from build123d import *

# Parameters (mm, degrees)
BOSS_EXTRUDE1_DEPTH = 6.35
SKETCH2_R           = 17.4625
SKETCH2_R_2         = 2.54
CUT_EXTRUDE1_DEPTH  = 706.764721773


with BuildPart() as part:
    # Sketch1 → Boss-Extrude1 (new body)
    with BuildSketch(Plane(origin=(0, 0, 0), x_dir=(0, 0, -1), z_dir=(1, 0, 0))):
        Polygon((0, 0), (0, 609.6), (50.8, 609.6), (355.6, 50.8), (355.6, 0), align=None)
        with BuildLine():
            Line((76.2, 101.6), (76.2, 357.336122773))
            ThreePointArc((76.2, 357.336122773), (95.323978482, 381.948549591), (123.898547552, 369.498966892))
            Line((123.898547552, 369.498966892), (263.390978155, 113.762844119))
            ThreePointArc((263.390978155, 113.762844119), (262.933861882, 88.634203469), (241.092430603, 76.2))
            Line((241.092430603, 76.2), (101.6, 76.2))
            ThreePointArc((101.6, 76.2), (83.639487758, 83.639487758), (76.2, 101.6))
        make_face(mode=Mode.SUBTRACT)
    extrude(amount=BOSS_EXTRUDE1_DEPTH)

    # Sketch2 → Cut-Extrude1 (cut, through all)
    with BuildSketch(Plane(origin=(6.35, 0, 0), x_dir=(0, 0, -1), z_dir=(1, 0, 0))):
        with Locations((25.4, 152.4)):
            Circle(SKETCH2_R)
        with Locations((25.4, 25.4)):
            Circle(SKETCH2_R_2)
        with Locations((76.2, 25.4)):
            Circle(SKETCH2_R_2)
        with Locations((127, 25.4)):
            Circle(SKETCH2_R_2)
        with Locations((177.8, 25.4)):
            Circle(SKETCH2_R_2)
        with Locations((228.6, 25.4)):
            Circle(SKETCH2_R_2)
        with Locations((279.4, 25.4)):
            Circle(SKETCH2_R_2)
        with Locations((25.4, 76.2)):
            Circle(SKETCH2_R_2)
        with Locations((330.2, 25.4)):
            Circle(SKETCH2_R_2)
        with Locations((25.4, 127)):
            Circle(SKETCH2_R_2)
        with Locations((25.4, 177.8)):
            Circle(SKETCH2_R_2)
        with Locations((25.4, 228.6)):
            Circle(SKETCH2_R_2)
        with Locations((25.4, 279.4)):
            Circle(SKETCH2_R_2)
        with Locations((25.4, 330.2)):
            Circle(SKETCH2_R_2)
        with Locations((25.4, 381)):
            Circle(SKETCH2_R_2)
        with Locations((25.4, 431.8)):
            Circle(SKETCH2_R_2)
        with Locations((25.4, 482.6)):
            Circle(SKETCH2_R_2)
        with Locations((25.4, 533.4)):
            Circle(SKETCH2_R_2)
        with Locations((25.4, 584.2)):
            Circle(SKETCH2_R_2)
    extrude(amount=-CUT_EXTRUDE1_DEPTH, mode=Mode.SUBTRACT)


solid = part.part
Design review of the part built by this model. Coordinates are the model's own, in mm. A direction names the side the tool comes from. Coordinates: 2 decimals unless noted, no trailing zeros. Loops run counter-clockwise (first coordinate to the right, second up) from the corner with the lowest first, then second, coordinate; pieces in that order, holes last. Notation, with made-up numbers: M -10,48.25 L 36,48.25 A26 cw 36,76.25 Z; hole C 89,-18 d9. An arc over 180 degrees is marked long. Answer as CSV lines item,"result".
Item 1: Add section A-A on x = 2.25. Count the separate pieces of the cut face and the enclosed holes in it, plus the area to 3 significant figures.
Answer list:
separate pieces,"1"
enclosed holes,"20"
area,"93,000 mm²"
Item 2: The part is to be moulded in two halves that separate along Y. For faces 1 (the face through (0, 241, -62)), 2 (the face through (3.131, 334.112, -201.066)), 3 (the face through (3.13, 243.42, -192.67)), say which applies: pulls with the +Y half, pulls with the -Y half, needs draft (parallel to the pull), parting line crosses it, or undercut.
Answer list:
face 1,"needs draft"
face 2,"pulls with the +Y half"
face 3,"undercut"
Item 3: Machinability: for faces 4 (the face through (6.35, 241, -62)), 5 (the face through (3.13, 83.44, -83.84)), which of the approach directions +Z, -Z, +X, -X, +Y, -Y give a long, thin tool a straight path to every point of the face, cutting with its end or side? Answer none if there is none.
Answer list:
face 4,"+Z, -Z, +X, +Y, -Y"
face 5,"+X, -X"
Item 4: Add section B-B on z = -107.5. State the section outline as (x, y) points, plus the area to 3 significant figures.
Answer list:
outline,"M 0,0 L 6.35,0 L 6.35,76.2 L 0,76.2 Z; M 0,382.04 L 6.35,382.04 L 6.35,505.65 L 0,505.65 Z"
area,"1,270 mm²"
Item 5: For P1, Ø1.5, axis at x = 1.5, y = 328.5, coming from the -Z side; P2, Ø1.9, axis at x = 3.5, z = -153, coming from the +Y side (3 decimals); P3, Ø1.5, axis at x = 5, z = -297, coming from the +Y side, all flat-tipped, find the tip position at first contact; note any pin that passes through.
Answer list:
P1,"z = -204.54"
P2,"y = 423.975"
P3,"y = 159.61"
Item 6: Add section C-C on y = 207.5. State the section outline as (x, z) points.
Answer list:
outline,"M 0,-270.13 L 6.35,-270.13 L 6.35,-212.26 L 0,-212.26 Z; M 0,-76.2 L 6.35,-76.2 L 6.35,0 L 0,0 Z"
Item 7: For probe 1 along Y at (x, z) = (4, -127); probe 2 along Y at (x, z) = (3.5, -177.8); probe 3 along Z at (x, y) = (5.25, 330.2), list the stretches that pass through material, from the lowest coordinate up.
Answer list:
probe 1,"0 to 22.86, 27.94 to 76.2, 363.81 to 469.9"
probe 2,"0 to 22.86, 27.94 to 76.2, 270.68 to 376.77"
probe 3,"-203.2 to -145.33, -76.2 to -27.94, -22.86 to 0"
